Here's how the part is built. I have some questions about the finished solid (model axes, mm). A direction names the side the tool comes from. Give positions to 0.01 mm unless a question says otherwise; leave off trailing zeros. Loops run counter-clockwise (first coordinate to the right, second up) from the corner with the lowest first, then second, coordinate; pieces in that order, holes last.
Q1. I need wall thicknesses on probe 1 along X at (y, z) = (0.55, 1.5); probe 2 along Y at (x, z) = (0, -0.9); probe 3 along Y at (x, z) = (0, 0.45). Which ranges of each line are inside material? Lowest first, please.
Q2. For faces 1 (the face through (0, 4, -0.725)), 2 (the face through (-2, 0, 0)), 3 (the face through (-1.45, 4, 0)), which set-ups out of +Z, -Z, +X, -X, +Y, -Y let a thin tool reach every point of the face, with its end or its side?
Q3. I'm going to push flat-ended pins straight in: P1, Ø1.4, axis at x = 0, z = -0.5, coming from the -Y side; P2, Ø0.6, axis at x = 3.5, y = 0.5, coming from the -Z side. Where does each tip first touch, or does it pass through?
Q4. Suppose I cut it at C-C (y = 1.9). List the corners of the cut face in (x, z) for me.
Q5. Suppose I cut it at A-A (y = 3.35). List the corners of the cut face in (x, z) for me (3 decimals), and give its area (3 significant figures).
Q6. Suppose I cut it at B-B (x = 0.5). List the corners of the cut face in (y, z) for me (3 decimals), and give its area (3 significant figures).
```python
from build123d import *

# Parameters (mm, degrees)
SKETCH1_W           = 6
SKETCH1_H           = 3.64
BOSS_EXTRUDE1_DEPTH = 3.25
SKETCH2_W           = 2.9
SKETCH2_H           = 1.45
BOSS_EXTRUDE2_DEPTH = 1
SKETCH3_W           = 0.5
SKETCH3_H           = 2
BOSS_EXTRUDE3_DEPTH = 0.2
FILLET1_R           = 0.1
SKETCH4_W           = 6.273612193
SKETCH4_H           = 3.809222638
SKETCH4_W_2         = 5.919575883
SKETCH4_H_2         = 3.566405206
CUT_EXTRUDE1_DEPTH  = 0.02
FILLET2_R           = 0.1
SKETCH5_W           = 1.8
SKETCH5_H           = 0.4
CUT_EXTRUDE2_DEPTH  = 5.02
BOSS_EXTRUDE4_START = -0.5
BOSS_EXTRUDE4_DEPTH = 1


# Read off the part's stored shape, not the designer's step: Boss-Extrude4
with BuildPart() as part:
    # Sketch1 → Boss-Extrude1 (new body)
    with BuildSketch(Plane(origin=(0, 0, 0), x_dir=(1, 0, 0), z_dir=(0, 1, 0))):
        Rectangle(SKETCH1_W, SKETCH1_H)
    extrude(amount=BOSS_EXTRUDE1_DEPTH)

    # Sketch2 → Boss-Extrude2 (add)
    with BuildSketch(Plane(origin=(0, 3.25, 0), x_dir=(1, 0, 0), z_dir=(0, 1, 0))):
        Rectangle(SKETCH2_W, SKETCH2_H)
    extrude(amount=BOSS_EXTRUDE2_DEPTH)

    # Sketch3 → Boss-Extrude3 (add)
    with BuildSketch(Plane(origin=(0, 3.25, 0), x_dir=(1, 0, 0), z_dir=(0, 1, 0))):
        with Locations((-2.45, 0)):
            Rectangle(SKETCH3_W, SKETCH3_H)
        with Locations((2.45, 0)):
            Rectangle(SKETCH3_W, SKETCH3_H)
    extrude(amount=BOSS_EXTRUDE3_DEPTH)

    # Fillet1
    fillet1_edges = [part.edges().sort_by_distance(p)[0] for p in [
        (-1.45, 3.75, -0.725),
        (-1.45, 3.75, 0.725),
        (1.45, 3.75, 0.725),
        (1.45, 3.75, -0.725),
        (-2.7, 3.35, -1),
        (-2.7, 3.35, 1),
        (-2.2, 3.35, 1),
        (-2.2, 3.35, -1),
        (2.2, 3.35, -1),
        (2.2, 3.35, 1),
        (2.7, 3.35, 1),
        (2.7, 3.35, -1),
    ]]
    fillet(fillet1_edges, radius=FILLET1_R)

    # Sketch4 → Cut-Extrude1 (cut)
    with BuildSketch(Plane(origin=(0, 3.15, 0), x_dir=(1, 0, 0), z_dir=(0, 1, 0))):
        with Locations((-0.037546102, -0.013653128)):
            Rectangle(SKETCH4_W, SKETCH4_H)
        with Locations((0.010712352, -0.001469434)):
            Rectangle(SKETCH4_W_2, SKETCH4_H_2, mode=Mode.SUBTRACT)
    extrude(amount=-CUT_EXTRUDE1_DEPTH, mode=Mode.SUBTRACT)

    # Fillet2
    fillet2_edges = [part.edges().sort_by_distance(p)[0] for p in [
        (-3, 1.565, -1.82),
        (3, 1.565, -1.82),
        (3, 1.565, 1.82),
        (-3, 1.565, 1.82),
        (-2.94907559, 3.14, -1.781733169),
        (2.970500293, 3.14, -1.781733169),
        (2.970500293, 3.14, 1.784672037),
        (-2.94907559, 3.14, 1.784672037),
        (-3, 3.2, -1.82),
        (3, 3.2, -1.82),
        (3, 3.2, 1.82),
        (-3, 3.2, 1.82),
    ]]
    fillet(fillet2_edges, radius=FILLET2_R)

    # Sketch5 → Cut-Extrude2 (cut)
    with BuildSketch(Plane(origin=(0, 0, -1.82), x_dir=(-1, 0, 0), z_dir=(0, 0, -1))):
        with Locations((0, 0.2)):
            Rectangle(SKETCH5_W, SKETCH5_H)
    extrude(amount=-CUT_EXTRUDE2_DEPTH, mode=Mode.SUBTRACT)

    # Boss-Extrude4 outline → Boss-Extrude4 (add)
    with BuildSketch(Plane.XY.offset(BOSS_EXTRUDE4_START)):
        with BuildLine():
            Line((4.173146956, -0.131659711), (4.173759731, -0.031661589))
            add(Edge.make_bspline(
                [(4.173759731, -0.031661589), (4.060884449, -0.030969905), (3.862308969, 0.050205488), (3.325841553, 0.329858602), (3.401409137, 1.062439588), (3, 1.211404175)],
                knots=[0, 0, 0, 0, 0.203003015, 0.331433955, 1, 1, 1, 1], degree=3))
            Line((3, 1.211404175), (3, 1.102542921))
            add(Edge.make_bspline(
                [(3, 1.102542921), (3.09279535, 1.055379151), (3.226381881, 0.869010627), (3.326243834, 0.475899683), (3.482197094, 0.170683307), (3.700920866, 0.013413394), (3.917304218, -0.082452634), (4.088231211, -0.131134455), (4.173146956, -0.131659711)],
                knots=[0.026799616, 0.026799616, 0.026799616, 0.026799616, 0.25, 0.5, 0.625, 0.75, 0.875, 1, 1, 1, 1], degree=3))
        make_face()
        with BuildLine():
            Line((-3, 1.102542921), (-3, 1.211404175))
            add(Edge.make_bspline(
                [(-3, 1.211404175), (-3.401409137, 1.062439588), (-3.325841553, 0.329858602), (-3.862308969, 0.050205488), (-4.060884449, -0.030969905), (-4.173759731, -0.031661589)],
                knots=[0, 0, 0, 0, 0.668566045, 0.796996985, 1, 1, 1, 1], degree=3))
            Line((-4.173759731, -0.031661589), (-4.173146956, -0.131659711))
            add(Edge.make_bspline(
                [(-4.173146956, -0.131659711), (-4.009862358, -0.125892663), (-3.668802958, -0.046437584), (-3.359459873, 0.383160744), (-3.261093668, 0.825417205), (-3.129401541, 1.021566363), (-3.02801046, 1.087631493), (-3.010284263, 1.097420299), (-3, 1.102542921)],
                knots=[0, 0, 0, 0, 0.25, 0.5, 0.75, 0.960893979, 0.976536388, 1, 1, 1, 1], degree=3))
        make_face()
    extrude(amount=BOSS_EXTRUDE4_DEPTH)


solid = part.part
```
Solutions:
1. probe 1: x = -3 to 3
1. probe 2: y = 0.4 to 3.25
1. probe 3: y = 0.4 to 4.25
2. face 1: -Z, +Y
2. face 2: +Z, -Z, -Y
2. face 3: +Z, -Z, +Y
3. P1: stops at y = 0.4
3. P2: stops at z = -0.5
4. outline: (-3, -1.72) arc R0.1 ccw to (-2.9, -1.82) - (2.9, -1.82) arc R0.1 ccw to (3, -1.72) - (3, 1.72) arc R0.1 ccw to (2.9, 1.82) - (-2.9, 1.82) arc R0.1 ccw to (-3, 1.72) - close
5. outline: (-2.7, -0.9) arc R0.1 ccw to (-2.6, -1) - (-2.3, -1) arc R0.1 ccw to (-2.2, -0.9) - (-2.2, 0.9) arc R0.1 ccw to (-2.3, 1) - (-2.6, 1) arc R0.1 ccw to (-2.7, 0.9) - close; (-1.45, -0.625) arc R0.1 ccw to (-1.35, -0.725) - (1.35, -0.725) arc R0.1 ccw to (1.45, -0.625) - (1.45, 0.625) arc R0.1 ccw to (1.35, 0.725) - (-1.35, 0.725) arc R0.1 ccw to (-1.45, 0.625) - close; (2.2, -0.9) arc R0.1 ccw to (2.3, -1) - (2.6, -1) arc R0.1 ccw to (2.7, -0.9) - (2.7, 0.9) arc R0.1 ccw to (2.6, 1) - (2.3, 1) arc R0.1 ccw to (2.2, 0.9) - close
5. area: 6.18 mm2
6. outline: (0.4, -1.82) - (3.13, -1.82) - (3.13, -1.782) - (3.15, -1.782) - (3.15, -1.82) - (3.25, -1.82) - (3.25, -0.725) - (4.25, -0.725) - (4.25, 0.725) - (3.25, 0.725) - (3.25, 1.82) - (3.15, 1.82) - (3.15, 1.785) - (3.13, 1.785) - (3.13, 1.82) - (0.4, 1.82) - close
6. area: 11.8 mm2
